from build123d import *

# Parameters (mm, degrees)
SKETCH_1_R      = 39.499995791
EXTRUDE_1_DEPTH = 10
EXTRUDE_2_DEPTH = 180


with BuildPart() as part:
    # 草图1 → 凸台-拉伸1 (new body)
    with BuildSketch(Plane.XY):
        Circle(SKETCH_1_R)
    extrude(amount=EXTRUDE_1_DEPTH)

    # 草图2 → 凸台-拉伸2 (add)
    with BuildSketch(Plane.XY.offset(10)):
        with BuildLine():
            Line((0, -69.800050309), (0, 39.499995791))
            ThreePointArc((0, 39.499995791), (-3.851829787, 39.3117422), (-7.666944594, 38.748775827))
            Line((-7.666944594, 38.748775827), (-7.666944594, -60.694122376))
            Line((-7.666944594, -60.694122376), (0, -69.800050309))
        make_face()
    extrude(amount=EXTRUDE_2_DEPTH)


solid = part.part
Can you work these out from the model? Positions are in its coordinate system, mm. A direction names the side the tool comes from. Coordinates: 2 decimals unless noted, no trailing zeros. Write each loop counter-clockwise with the first axis right and the second up, starting at its lowest first coordinate (ties: lowest second). Pieces come first, ordered by that corner, then holes. Notation, with made-up numbers: (61.5, -17.75) -> (102.5, -17.75) arc R22 ccw to (102.5, 21.25) -> close; hole circle Ø9 at (57, 26). An arc over 180 degrees is marked (long way). Answer as CSV lines item,"result".
1) Will these pins go through, and if not, where does the flat tip stop? P1, Ø1, axis at x = -28, y = -28, coming from the +Z side; P2, Ø6, axis at y = -37.5, z = 161.5, coming from the +X side; P3, Ø3, axis at x = -4, z = 133, coming from the -Y side.
Check result:
P1,"z = 10"
P2,"x = 0"
P3,"y = -66.83"
2) If we section it at D-D on y = -28.5: Please give me the cut outline in (x, z).
Check result:
outline,"(-27.35, 0) -> (27.35, 0) -> (27.35, 10) -> (0, 10) -> (0, 190) -> (-7.67, 190) -> (-7.67, 10) -> (-27.35, 10) -> close"
3) If I drill on line 1 (X direction, y = -33.5, z = 103); line 2 (Z direction, x = -25.5, y = 14.5), over which ranges is the centre line in solid material (lowest first)? Write a range as from..to.
Check result:
line 1,"-7.67..0"
line 2,"0..10"
4) On a 3-axis mill with a long thin cutter (end or side, diameter ignored), from which of +Z, -Z, +X, -X, +Y, -Y can I reach the whole of each face in a straight line? I mean faces 1 (the flat face through (-7.667, -10, 99)), 2 (the flat face through (15, 1, 10)), 3 (the flat face through (-3.89, -65.18, 98.74)). Say none if no direction works.
Check result:
face 1,"+Z, -X, +Y, -Y"
face 2,"+Z, +X, +Y, -Y"
face 3,"+Z, -Z, -X, -Y"
5) If we section it at B-B on z = 86.5: Please give me the cut outline in (x, y).
Check result:
outline,"(-7.67, -60.69) -> (0, -69.8) -> (0, 39.5) arc R39.5 ccw to (-7.67, 38.75) -> close"
6) If we section it at A-A on y = 0: Please give me the cut outline in (x, z), then the cut area to 3 significant figures.
Check result:
outline,"(-39.5, 0) -> (39.5, 0) -> (39.5, 10) -> (0, 10) -> (0, 190) -> (-7.67, 190) -> (-7.67, 10) -> (-39.5, 10) -> close"
area,"2,170 mm²"
7) If we section it at C-C on x = -16: Please give me the cut outline in (y, z), then the cut area to 3 significant figures.
Check result:
outline,"(-36.11, 0) -> (36.11, 0) -> (36.11, 10) -> (-36.11, 10) -> close"
area,"722 mm²"
